from build123d import *

# Parameters (mm, degrees)
SKETCH_2_W = 0.5
SKETCH_2_H = 2.5


with BuildPart() as part:
    # ｽｹｯﾁ1 → 回転1 (revolve)
    with BuildSketch(Plane(origin=(0, 0, 0), x_dir=(0, 0, -1), z_dir=(1, 0, 0)), mode=Mode.PRIVATE) as revolve_1_sk:
        Polygon((0, 7.5), (5, 7.5), (5, 13), (3.9, 13), (3.9, 12), (0, 12), align=None)
    revolve(revolve_1_sk.sketch.rotate(Axis((0, 0, 0), (0, 0, -1)), 90), axis=Axis((0, 0, 0), (0, 0, -1)))

    # ｽｹｯﾁ2 → ｶｯﾄ - 回転1 (revolve, cut)
    with BuildSketch(Plane(origin=(0, 0, 0), x_dir=(0, 0, -1), z_dir=(1, 0, 0)), mode=Mode.PRIVATE) as cut_revolve_1_sk:
        with Locations((0.25, 9.75)):
            Rectangle(SKETCH_2_W, SKETCH_2_H)
        with Locations((4.75, 9.75)):
            Rectangle(SKETCH_2_W, SKETCH_2_H)
    revolve(cut_revolve_1_sk.sketch.rotate(Axis((0, 0, 0), (0, 0, -1)), 90), axis=Axis((0, 0, 0), (0, 0, -1)), mode=Mode.SUBTRACT)


solid = part.part
Design review of the part built by this model. Coordinates are the model's own, in mm. A direction names the side the tool comes from. Round coordinates to 2 decimals unless told otherwise and drop trailing zeros. Loops run counter-clockwise (first coordinate to the right, second up) from the corner with the lowest first, then second, coordinate; pieces in that order, holes last. Notation, with made-up numbers: (43.5, 16) - (55.5, 16) arc R6 ccw to (55.5, 20) - close; hole circle Ø7 at (-13, -1). An arc over 180 degrees is marked (long way). One line per item, written item: value. Start each with the question number.
1) Insertion check: pin 1 Ø3 at (x, z) = (-7, -2) entering from -Y; pin 2 Ø1.5 at (y, z) = (0.5, -0.5) entering from -X; pin 3 Ø1.5 at (x, z) = (-4, -2) entering from -Y. Each pin has a flat end and moves straight along its axis. Give the tip position at first contact, or say it passes through.
2) For faces 1 (the cylindrical face through (4.032, -6.324, -2.535)), 2 (the cylindrical face through (-1.107, -8.428, -4.754)), 3 (the flat face through (-3.2, 8.1, -0.5)), list the 3-axis set-ups (+Z, -Z, +X, -X, +Y, -Y) from which the entire face can be reached by the end or side of a thin tool; tool diameter is ignored.
3) To check wall thickness, follow L1, parallel to Y at x = 0, z = -0.3; L2, parallel to Y at x = 0, z = -4.7; L3, parallel to Y at x = 0, z = -2.25. State the ranges of each line that lie inside material, in increasing order. Write a range as from..to.
4) Consider section A-A on x = 0. Give the boundary of the cut face in (y, z).
5) Consider section C-C on z = -3. Give the boundary of the cut face in (x, y), then the cut area to 3 significant figures.
6) Draft analysis for pull direction Y (two halves, no side actions). For faces 4 (the cylindrical face through (-2.38, 10.74, -4.75)), 5 (the cylindrical face through (11.446, -3.604, -1.923)), 6 (the flat face through (-3.2, 8.1, -4.5)), 7 (the flat face through (0, 8, 0)), state which applies: +Y half, -Y half, draft (parallel to the pull), parting line (faces both ways), or undercut.
7) Consider section D-D on x = 9.5. Give the boundary of the cut face in (y, z).
Reported:
1. pin 1: stops at y = -10.67
1. pin 2: stops at x = -12
1. pin 3: stops at y = -11.55
2. face 1: +Z, -Z
2. face 2: -Z
2. face 3: +Z
3. L1: y = -12..-11, -8.5..-7.5, 7.5..8.5, 11..12
3. L2: y = -13..-11, -8.5..-7.5, 7.5..8.5, 11..13
3. L3: y = -12..-7.5, 7.5..12
4. outline: (-13, -5) - (-11, -5) - (-11, -4.5) - (-8.5, -4.5) - (-8.5, -5) - (-7.5, -5) - (-7.5, 0) - (-8.5, 0) - (-8.5, -0.5) - (-11, -0.5) - (-11, 0) - (-12, 0) - (-12, -3.9) - (-13, -3.9) - close; (7.5, -5) - (8.5, -5) - (8.5, -4.5) - (11, -4.5) - (11, -5) - (13, -5) - (13, -3.9) - (12, -3.9) - (12, 0) - (11, 0) - (11, -0.5) - (8.5, -0.5) - (8.5, 0) - (7.5, 0) - close
5. outline: circle Ø24 at (0, 0); hole circle Ø15 at (0, 0)
5. area: 276 mm^2
6. face 4: undercut
6. face 5: parting line
6. face 6: undercut
6. face 7: draft
7. outline: (-8.87, -5) - (-5.55, -5) - (-5.55, -4.5) - (5.55, -4.5) - (5.55, -5) - (8.87, -5) - (8.87, -3.9) - (7.33, -3.9) - (7.33, 0) - (5.55, 0) - (5.55, -0.5) - (-5.55, -0.5) - (-5.55, 0) - (-7.33, 0) - (-7.33, -3.9) - (-8.87, -3.9) - close
